Design review of the part shown in the three views and the two pictorial views. Dimensions are in mm from the part's minimum x, y and z. A direction names the side the tool comes from. Coordinates: 2 decimals unless noted, no trailing zeros. Loops run counter-clockwise (first coordinate to the right, second up) from the corner with the lowest first, then second, coordinate; pieces in that order, holes last. Notation, with made-up numbers: (-37, 12.25) -> (15, 12.25) arc R10 ccw to (15, 30.25) -> close; hole circle Ø10 at (12.5, 86). An arc over 180 degrees is marked (long way). Use a Markdown table: item, result. Add a question column.
Q1. For the marked faces 1, 2 and 3, list the 3-axis set-ups (+Z, -Z, +X, -X, +Y, -Y) from which the entire face can be reached by the end or side of a thin tool; tool diameter is ignored.
Q2. Clearance check with flat-ended pins moving along their axes: pin 1 Ø1.5 at (x, z) = (9, 14) entering from +Y; pin 2 Ø12.5 at (x, z) = (22.5, 26.5) entering from +Y; pin 3 Ø3 at (x, z) = (31.5, 15) entering from +Y; pin 4 Ø4 at (x, y) = (22.5, 56) entering from -Z. State where each tip first meets the part, or that it passes through.
Q3. Take a section at D-D on x = 33.5. Write out the cut boundary in (y, z), plus the area to 3 significant figures.
Q4. Take a section at A-A on x = 16.5. Write out the cut boundary in (y, z), plus the area to 3 significant figures.
Q5. Draft analysis for pull direction Y (two halves, no side actions). For the marked faces 4, 5 and 6, state which applies: pulls with the +Y half, pulls with the -Y half, needs draft (parallel to the pull), parting line crosses it, or undercut.
Q6. Take a section at B-B on y = 5. Write out the cut boundary in (x, z).
Q7. For probe 1 along Y at (x, z) = (26, 38); probe 2 along Y at (x, z) = (25, 16); probe 3 along Z at (x, y) = (37.5, 32.5) (1 decimal), list the stretches that pass through material, from the lowest coordinate up.
Q8. Take a section at C-C on z = 11.5. Write out the cut boundary in (x, y).
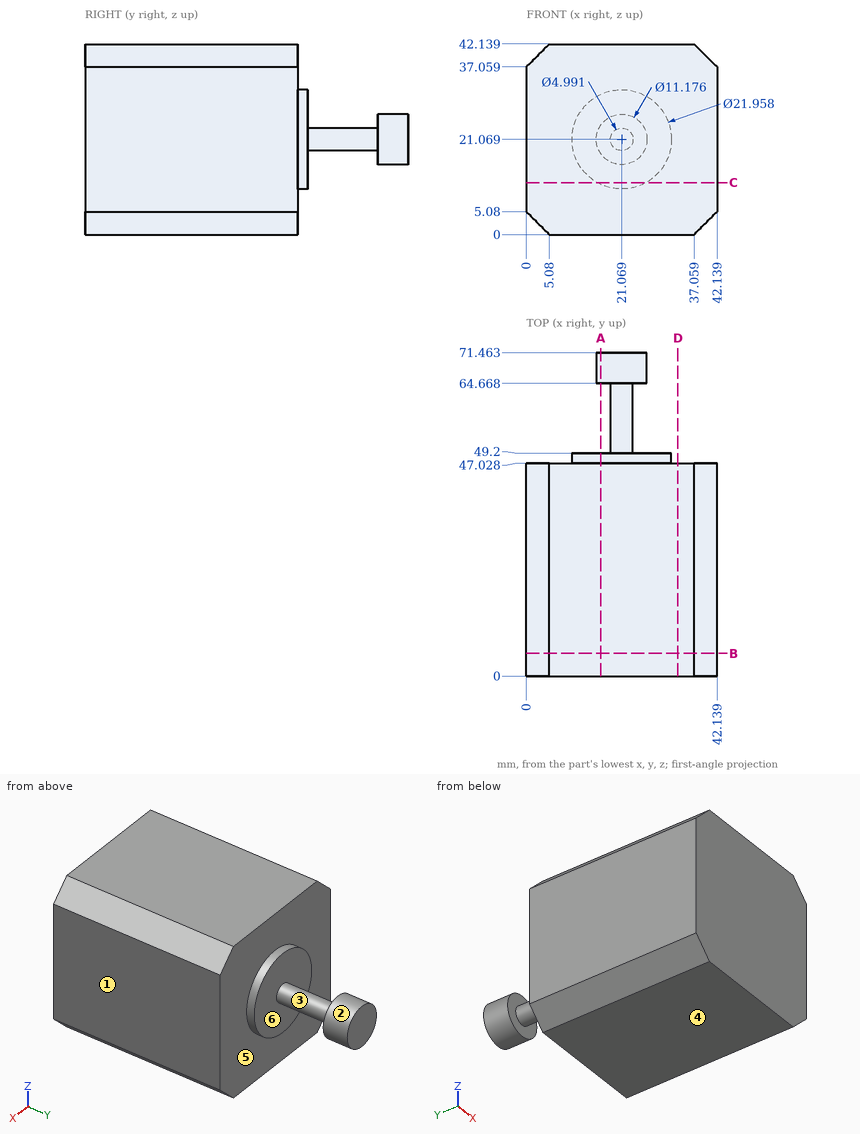
Answer list:
| question | item | result |
|---|---|---|
| 1 | face 1 | +Z, -Z, +X, +Y, -Y |
| 1 | face 2 | +Y |
| 1 | face 3 | none |
| 2 | pin 1 | y = 47.03 |
| 2 | pin 2 | y = 71.46 |
| 2 | pin 3 | y = 49.2 |
| 2 | pin 4 | z = 18.57 |
| 3 | outline | (0, 0) -> (47.03, 0) -> (47.03, 42.14) -> (0, 42.14) -> close |
| 3 | area | 1,980 mm² |
| 4 | outline | (0, 0) -> (47.03, 0) -> (47.03, 11.09) -> (49.2, 11.09) -> (49.2, 31.05) -> (47.03, 31.05) -> (47.03, 42.14) -> (0, 42.14) -> close; (64.67, 17.85) -> (71.46, 17.85) -> (71.46, 24.29) -> (64.67, 24.29) -> close |
| 4 | area | 2,070 mm² |
| 5 | face 4 | needs draft |
| 5 | face 5 | pulls with the +Y half |
| 5 | face 6 | undercut |
| 6 | outline | (0, 5.08) -> (5.08, 0) -> (37.06, 0) -> (42.14, 5.08) -> (42.14, 37.06) -> (37.06, 42.14) -> (5.08, 42.14) -> (0, 37.06) -> close |
| 7 | probe 1 | 0 to 47.03 |
| 7 | probe 2 | 0 to 49.2 |
| 7 | probe 3 | 0.4 to 41.7 |
| 8 | outline | (0, 0) -> (42.14, 0) -> (42.14, 47.03) -> (26.45, 47.03) -> (26.45, 49.2) -> (15.69, 49.2) -> (15.69, 47.03) -> (0, 47.03) -> close |
